Verification items for the finished model (mm, model axes). Give positions to 0.01 mm unless a question says otherwise; leave off trailing zeros. Loops run counter-clockwise (first coordinate to the right, second up) from the corner with the lowest first, then second, coordinate; pieces in that order, holes last. Notation, with made-up numbers: M 70,39.5 L 115,39.5 A21 cw 115,72.5 Z; hole C -6,-32 d7. An arc over 180 degrees is marked long. Put each result on its own line as item: value. Start each with the question number.
from build123d import *

# Parameters (mm, degrees)
SKETCH_1_R      = 1.6
EXTRUDE_1_DEPTH = 5
FILLET_1_R      = 2


with BuildPart() as part:
    # 草图1 → 凸台-拉伸1 (new body)
    with BuildSketch(Plane(origin=(0, 0, 0), x_dir=(1, 0, 0), z_dir=(0, 1, 0))):
        with BuildLine():
            Line((-13.5, 2.5), (13.5, 2.5))
            Line((13.5, 2.5), (42.477774789, 10.264571353))
            Line((42.477774789, 10.264571353), (43.176188432, 7.65805615))
            Line((43.176188432, 7.65805615), (43.176188432, 5.529700605))
            Line((43.176188432, 5.529700605), (41.964432742, 7.37098368))
            Line((41.964432742, 7.37098368), (41.964432742, 5.242628135))
            Line((41.964432742, 5.242628135), (40.960741016, 7.044242108))
            Line((40.960741016, 7.044242108), (40.960741016, 4.915886563))
            Line((40.960741016, 4.915886563), (39.95704929, 6.717500536))
            Line((39.95704929, 6.717500536), (39.95704929, 4.589144991))
            Line((39.95704929, 4.589144991), (38.953357563, 6.390758965))
            Line((38.953357563, 6.390758965), (39.000927635, 4.332952966))
            Line((39.000927635, 4.332952966), (38.334050279, 4.154263717))
            ThreePointArc((38.334050279, 4.154263717), (28.290848144, 3.559013712), (19.295554958, -0.947085729))
            Line((19.295554958, -0.947085729), (13.5, -2.5))
            Line((13.5, -2.5), (-13.5, -2.5))
            Line((-13.5, -2.5), (-13.5, 2.5))
        make_face()
        with Locations(Location((-11, 0, 0), (0, 0, 270))):
            Circle(SKETCH_1_R, mode=Mode.SUBTRACT)
        with Locations(Location((11, 0, 0), (0, 0, 90))):
            Circle(SKETCH_1_R, mode=Mode.SUBTRACT)
    extrude(amount=EXTRUDE_1_DEPTH)

    # 圆角1
    fillet_1_edges = [part.edges().sort_by_distance(p)[0] for p in [
        (13.5, 2.5, 2.5),
        (-13.5, 2.5, 2.5),
        (-13.5, 2.5, -2.5),
        (13.5, 2.5, -2.5),
        (42.477774789, 2.5, -10.264571353),
        (38.334050279, 2.5, -4.154263717),
        (19.295554958, 2.5, 0.947085729),
    ]]
    fillet(fillet_1_edges, radius=FILLET_1_R)


solid = part.part
Q1. Cross-section at A-A, the plane x = 11. Record the boundary of the cut face in (y, z).
Q2. Cross-section at B-B, the plane y = 1.5. Record the boundary of the cut face in (x, z), then the cut area to 3 significant figures.
Q3. Cross-section at D-D, the plane x = 27.5. Record the boundary of the cut face in (y, z), then the cut area to 3 significant figures.
Q4. Release check for a two-part mould opening along X. For faces 1 (the face through (-13.5, 2, 0)), 2 (the face through (39.957, 2, -6)), 3 (the face through (1, 2, -2.5)) record: pulls with the +X half, pulls with the -X half, needs draft (parallel to the pull), parting line crosses it, or undercut.
Q5. Cross-section at C-C, the plane z = 0. Record the boundary of the cut face in (x, y).
Q6. Go/stop test with flat-tipped pins: pin 1 (3 mm diameter, centred on x = -11, z = 0, fed in from -Y); pin 2 (3 mm diameter, centred on y = 3.5, z = 0, fed in from +X). Record where each tip stops, or that it passes through.
Q7. Scan lines: L1, parallel to Z at x = 11, y = 3.15; L2, parallel to X at y = 3.55, z = 0; L3, parallel to X at y = 3.65, z = -0.5. Record each from-to range of solid material in increasing order.
Ans:
1. outline: M 0,-2.5 L 5,-2.5 L 5,-1.6 L 0,-1.6 Z; M 0,1.6 L 5,1.6 L 5,2.5 L 0,2.5 Z
2. outline: M -13.5,-0.5 A2 ccw -11.5,-2.5 L 13.24,-2.5 A2 cw 13.75,-2.57 L 40.55,-9.75 A2 ccw 43,-8.33 L 43.18,-7.66 L 43.18,-5.53 L 41.96,-7.37 L 41.96,-5.24 L 40.96,-7.04 L 40.96,-4.92 L 39.96,-6.72 L 39.96,-4.59 L 38.95,-6.39 L 39,-4.33 L 38.72,-4.26 A2 ccw 37.95,-4.21 A25 cw 19.6,0.71 A2 ccw 18.91,1.05 L 13.75,2.43 A2 ccw 13.24,2.5 L -11.5,2.5 A2 ccw -13.5,0.5 Z; hole C -11,0 d3.2; hole C 11,0 d3.2
2. area: 232 mm^2
3. outline: M 0,-6.25 L 5,-6.25 L 5,-3.33 L 0,-3.33 Z
3. area: 14.6 mm^2
4. face 1: pulls with the -X half
4. face 2: undercut
4. face 3: needs draft
5. outline: M -13.5,0 L -12.6,0 L -12.6,5 L -13.5,5 Z; M -9.4,0 L 9.4,0 L 9.4,5 L -9.4,5 Z; M 12.6,0 L 20.58,0 L 20.58,5 L 12.6,5 Z
6. pin 1: passes through
6. pin 2: stops at x = 23.05
7. L1: z = -2.5 to -1.6, 1.6 to 2.5
7. L2: x = -13.5 to -12.6, -9.4 to 9.4, 12.6 to 20.58
7. L3: x = -13.5 to -12.52, -9.48 to 9.48, 12.52 to 21.34
